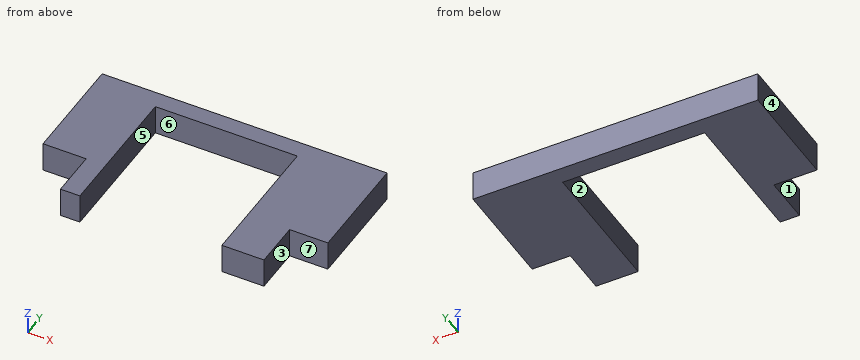
```python
from build123d import *

# Parameters (mm, degrees)
BOSS_EXTRUDE1_DEPTH = 3.175


with BuildPart() as part:
    # Sketch1 → Boss-Extrude1 (new body)
    with BuildSketch(Plane.XY):
        Polygon((0, 16.66), (30.1, 16.66), (30.1, 6.34), (30.1, 5.14), (26.06, 5.14), (26.06, 0.14), (25.36, 0.14), (21.61, 0.14), (21.61, 5.14), (21.61, 6.34), (21.61, 14.84), (6.61, 14.84), (6.61, 6.34), (6.61, 5.14), (6.61, 0.14), (4.559999976, 0.14), (4.559999976, 5.14), (0, 5.14), (0, 6.34), align=None)
    extrude(amount=-BOSS_EXTRUDE1_DEPTH)


solid = part.part
```
Geometry check sheet. Reference: the model listing, model coordinates, mm. Face numbers are marked on the shaded views. A direction names the side the tool comes from. Give positions to 0.01 mm unless a question says otherwise; leave off trailing zeros. Write each loop counter-clockwise with the first axis right and the second up, starting at its lowest first coordinate (ties: lowest second). Pieces come first, ordered by that corner, then holes. Notation, with made-up numbers: (-14.5, 29) - (-6.5, 29) arc R26 cw to (-6.5, 50) - close; hole circle Ø5 at (63, 17). An arc over 180 degrees is marked (long way). Use a Markdown table: item, result.
Q1. Section check D-D, the plane x = 2. Enter the section's corners in (y, z) (3 decimals).
Computed:
| item | result |
|---|---|
| outline | (5.14, -3.175) - (16.66, -3.175) - (16.66, 0) - (5.14, 0) - close |
Q2. Set-up check for the marked faces 1, 2 and 3: record each of +Z, -Z, +X, -X, +Y, -Y from which the full face is reachable in a straight line by a thin tool's end or side.
Computed:
| item | result |
|---|---|
| face 1 | +Z, -Z, -X, -Y |
| face 2 | +Z, -Z, -Y |
| face 3 | +Z, -Z, +X, -Y |
Q3. Section check B-B, the plane z = -0.6. Enter the section's corners in (x, y), then the cut area to 3 significant figures.
Computed:
| item | result |
|---|---|
| outline | (0, 5.14) - (4.56, 5.14) - (4.56, 0.14) - (6.61, 0.14) - (6.61, 14.84) - (21.61, 14.84) - (21.61, 0.14) - (26.06, 0.14) - (26.06, 5.14) - (30.1, 5.14) - (30.1, 16.66) - (0, 16.66) - close |
| area | 234 mm² |
Q4. Go/stop test with flat-tipped pins: P1, Ø1, axis at x = 7.5, z = -1, coming from the -Y side; P2, Ø1, axis at x = 27.5, z = -2, coming from the -Y side; P3, Ø3, axis at x = 15, y = 12.5, coming from the +Z side; P4, Ø1.6, axis at y = 3.5, z = -2, coming from the -X side. Record where each tip stops, or that it passes through.
Computed:
| item | result |
|---|---|
| P1 | stops at y = 14.84 |
| P2 | stops at y = 5.14 |
| P3 | passes through |
| P4 | stops at x = 4.56 |
Q5. Thickness scan on L1, parallel to X at y = 10.25, z = -1.2; L2, parallel to X at y = 1.5, z = -2.4; L3, parallel to Y at x = 14.5, z = -1.6. Record the ranges inside material, lowest first. Write a range as [from, to].
Computed:
| item | result |
|---|---|
| L1 | x = [0, 6.61], [21.61, 30.1] |
| L2 | x = [4.56, 6.61], [21.61, 26.06] |
| L3 | y = [14.84, 16.66] |
Q6. Section check A-A, the plane y = 14.5. Enter the section's corners in (x, z) (3 decimals), then the cut area to 3 significant figures.
Computed:
| item | result |
|---|---|
| outline | (0, -3.175) - (6.61, -3.175) - (6.61, 0) - (0, 0) - close; (21.61, -3.175) - (30.1, -3.175) - (30.1, 0) - (21.61, 0) - close |
| area | 47.9 mm² |
Q7. Draft check along X on the marked faces 4, 5, 6 and 7. Enter one of: pulls with the +X half, pulls with the -X half, needs draft (parallel to the pull), parting line crosses it, or undercut.
Computed:
| item | result |
|---|---|
| face 4 | pulls with the -X half |
| face 5 | undercut |
| face 6 | undercut |
| face 7 | needs draft |
Q8. Section check C-C, the plane y = 4.25. Enter the section's corners in (x, z) (3 decimals), then the cut area to 3 significant figures.
Computed:
| item | result |
|---|---|
| outline | (4.56, -3.175) - (6.61, -3.175) - (6.61, 0) - (4.56, 0) - close; (21.61, -3.175) - (26.06, -3.175) - (26.06, 0) - (21.61, 0) - close |
| area | 20.6 mm² |
